Part model, mm, in its own coordinate system. A direction names the side the tool comes from. Round coordinates to 2 decimals unless told otherwise and drop trailing zeros. Loops run counter-clockwise (first coordinate to the right, second up) from the corner with the lowest first, then second, coordinate; pieces in that order, holes last. Notation, with made-up numbers: (-18.5, 56.25) -> (-12.5, 56.25) arc R23 ccw to (-12.5, 79.25) -> close; hole circle Ø8 at (35.25, 53.25). An arc over 180 degrees is marked (long way). Answer as CSV lines item,"result".
from build123d import *

# Parameters (mm, degrees)
F0_W      = 30
F0_H      = 15
F1_DEPTH  = 46
F2_R      = 1.25
F3_DEPTH  = 46
F4_W      = 24
F4_H      = 40
F5_DEPTH  = 12
F6_R      = 3
F7_DEPTH  = 12
F8_W      = 30
F8_H      = 3
F9_DEPTH  = 46.001
F10_R     = 1.3
F11_DEPTH = 10


with BuildPart() as f1:
    # F0 (on Front) → F1 (new body)
    with BuildSketch(Plane.XZ):
        Rectangle(F0_W, F0_H)
    extrude(amount=F1_DEPTH)

    # F2 (on face) → F3 (cut, through all)
    with BuildSketch(Plane.XZ.offset(46)):
        with Locations((-7.5, 0)):
            Circle(F2_R)
        with Locations((7.5, 0)):
            Circle(F2_R)
    extrude(amount=-F3_DEPTH, mode=Mode.SUBTRACT)

    # F4 (on face) → F5 (cut)
    with BuildSketch(Plane.XY.offset(7.5)):
        with Locations((0, -23)):
            Rectangle(F4_W, F4_H)
    extrude(amount=-F5_DEPTH, mode=Mode.SUBTRACT)

    # F6 (on face) → F7 (join)
    with BuildSketch(Plane.XY.offset(-4.5)):
        with Locations((0, -3)):
            Circle(F6_R)
        with Locations((0, -43)):
            Circle(F6_R)
    extrude(amount=F7_DEPTH)

    # F8 (on face) → F9 (cut, through all)
    with BuildSketch(Plane(origin=(0, 0, 0), x_dir=(-1, 0, 0), z_dir=(0, 1, 0))):
        with Locations((0, 6)):
            Rectangle(F8_W, F8_H)
    extrude(amount=-F9_DEPTH, mode=Mode.SUBTRACT)

    # F10 (on face) → F11 (cut)
    with BuildSketch(Plane.XY.offset(4.5)):
        with Locations((0, -3)):
            Circle(F10_R)
        with Locations((0, -43)):
            Circle(F10_R)
    extrude(amount=-F11_DEPTH, mode=Mode.SUBTRACT)


solid = f1.part
Q1. Saw through at A-A, the plane x = -7.5. Write the cut outline in (y, z).
Geometry results:
outline,"(-46, -7.5) -> (0, -7.5) -> (0, -1.25) -> (-3, -1.25) -> (-3, -4.5) -> (-43, -4.5) -> (-43, -1.25) -> (-46, -1.25) -> close; (-46, 1.25) -> (-43, 1.25) -> (-43, 4.5) -> (-46, 4.5) -> close; (-3, 1.25) -> (0, 1.25) -> (0, 4.5) -> (-3, 4.5) -> close"
Q2. Drill centre lines: line 1 along X through (y, z) = (-8, 4); line 2 along Y through (x, z) = (5, 3.75); line 3 along X through (y, z) = (-3.5, -3.75). Where is each one in solid material? Low to high.
Geometry results:
line 1,"-15 to -12, 12 to 15"
line 2,"-46 to -43, -3 to 0"
line 3,"-15 to -12, -2.96 to -1.2, 1.2 to 2.96, 12 to 15"
Q3. Drop flat-ended pins along their axis: P1, Ø1.5, axis at x = 0.5, y = -26, coming from the +Z side; P2, Ø1.5, axis at x = 7.5, z = 0, coming from the +Y side; P3, Ø2.5, axis at x = 0, y = -43, coming from the +Z side. Give the stop position or say it passes through.
Geometry results:
P1,"z = -4.5"
P2,"through"
P3,"z = -5.5"
Q4. Saw through at B-B, the plane y = -38. Write the cut outline in (x, z).
Geometry results:
outline,"(-15, -7.5) -> (15, -7.5) -> (15, 4.5) -> (12, 4.5) -> (12, -4.5) -> (-12, -4.5) -> (-12, 4.5) -> (-15, 4.5) -> close"
Q5. Saw through at D-D, the plane x = 0. Write the cut outline in (y, z), then the cut area to 3 significant figures.
Geometry results:
outline,"(-46, -7.5) -> (0, -7.5) -> (0, 4.5) -> (-1.7, 4.5) -> (-1.7, -5.5) -> (-4.3, -5.5) -> (-4.3, 4.5) -> (-6, 4.5) -> (-6, -4.5) -> (-40, -4.5) -> (-40, 4.5) -> (-41.7, 4.5) -> (-41.7, -5.5) -> (-44.3, -5.5) -> (-44.3, 4.5) -> (-46, 4.5) -> close"
area,"194 mm2"
Q6. Which spindle directions (+Z, -Z, +X, -X, +Y, -Y) get a long thin tool onto all of the face, cutting with end or side? Do faces 1 (the face through (-8.75, -44.52, 0.05)), 2 (the face through (0, -40, 0)). Say none if no direction does.
Geometry results:
face 1,"+Y, -Y"
face 2,"+Z"
Q7. Saw through at C-C, the plane z = -3.5. Write the cut outline in (x, y), then the cut area to 3 significant figures.
Geometry results:
outline,"(-15, -46) -> (15, -46) -> (15, 0) -> (-15, 0) -> close; hole (-12, -43) -> (-3, -43) arc R3 cw to (3, -43) -> (12, -43) -> (12, -3) -> (3, -3) arc R3 cw to (-3, -3) -> (-12, -3) -> close; hole circle Ø2.6 at (0, -43); hole circle Ø2.6 at (0, -3)"
area,"438 mm2"
Q8. Two-plate mould, pull along Y, no slides. Class faces 3 (the face through (6.25, -44.52, 0.05)), 4 (the face through (0, -23, -4.5)), 5 (the face through (0, 0, -1)): pulls with the +Y half, pulls with the -Y half, needs draft (parallel to the pull), parting line crosses it, or undercut.
Geometry results:
face 3,"needs draft"
face 4,"undercut"
face 5,"pulls with the +Y half"
